The drawing under review shows one solid part. Ordinate dimensions are in mm from its lowest x, y, z. Give positions to 0.01 mm unless a question says otherwise; leave off trailing zeros. Write each loop counter-clockwise with the first axis right and the second up, starting at its lowest first coordinate (ties: lowest second). Pieces come first, ordered by that corner, then holes. Notation, with made-up numbers: M 77,77 L 85,77 A20 ccw 85,98 Z; hole C 12.25,5.5 d10. An arc over 180 degrees is marked long. Answer as a JSON object with one key per item and string values. Group by question number.
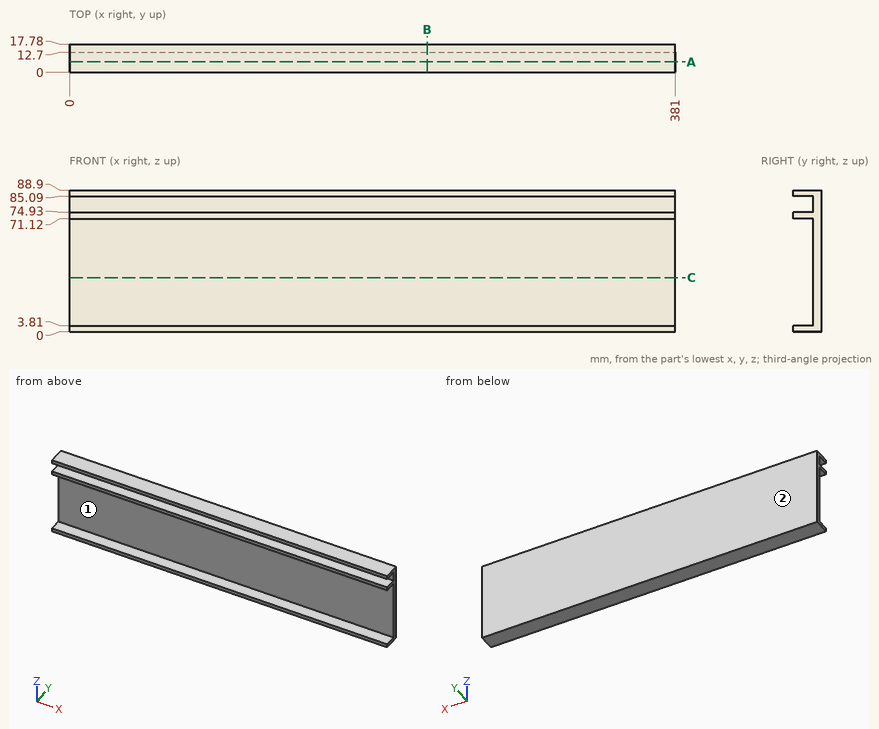
Item 1: Consider section B-B (x = 225). Give the boundary of the cut face in (y, z).
Item 2: Consider section C-C (z = 34). Give the boundary of the cut face in (x, y), plus the area to 3 significant figures.
Item 3: To check wall thickness, follow probe 1 along Z at (x, y) = (113, 10); probe 2 along Y at (x, z) = (72, 47). State the ranges of each line that lie inside material, in increasing order.
Item 4: Insertion check: P1, Ø5, axis at x = 202.5, z = 40, coming from the -Y side; P2, Ø10, axis at x = 170.5, y = 6, coming from the -Z side. Each pin has a flat end and moves straight along its axis. Give the tip position at first contact, or say it passes through.
Item 5: Consider section A-A (y = 6.5). Give the boundary of the cut face in (x, z), plus the area to 3 significant figures.
Item 6: Draft analysis for pull direction Z (two halves, no side actions). For the marked faces 1 and 2, state which applies: released by +Z, released by -Z, zero draft, split by the parting line, or undercut.
Result set:
{
 "1": {"outline": "M 0,0 L 17.78,0 L 17.78,88.9 L 0,88.9 L 0,85.09 L 12.7,85.09 L 12.7,74.93 L 0,74.93 L 0,71.12 L 12.7,71.12 L 12.7,3.81 L 0,3.81 Z"},
 "2": {"outline": "M 0,12.7 L 381,12.7 L 381,17.78 L 0,17.78 Z", "area": "1,940 mm^2"},
 "3": {"probe 1": "z = 0 to 3.81, 71.12 to 74.93, 85.09 to 88.9", "probe 2": "y = 12.7 to 17.78"},
 "4": {"P1": "stops at y = 12.7", "P2": "stops at z = 0"},
 "5": {"outline": "M 0,0 L 381,0 L 381,3.81 L 0,3.81 Z; M 0,71.12 L 381,71.12 L 381,74.93 L 0,74.93 Z; M 0,85.09 L 381,85.09 L 381,88.9 L 0,88.9 Z", "area": "4,350 mm^2"},
 "6": {"face 1": "undercut", "face 2": "zero draft"}
}
